Geometry check sheet. Reference: drawing and pictorial views, mm from the part's lowest x, y, z. Round coordinates to 2 decimals unless told otherwise and drop trailing zeros. Loops run counter-clockwise (first coordinate to the right, second up) from the corner with the lowest first, then second, coordinate; pieces in that order, holes last. Notation, with made-up numbers: (31, -1.5) - (70, -1.5) arc R16 cw to (70, 10.5) - close; hole circle Ø8 at (72, 68.25). An arc over 180 degrees is marked (long way). Answer as CSV lines item,"result". Start each with the question number.
1) Cross-section at D-D on y = 5.5. Record the boundary of the cut face in (x, z), and give its area (3 significant figures).
2) Draft check along X on the marked faces 1, 2 and 3. Enter one of: released by +X, released by -X, zero draft, split by the parting line, or undercut.
3) Cross-section at C-C on y = 3.25. Record the boundary of the cut face in (x, z).
4) Cross-section at B-B on z = 0.6. Record the boundary of the cut face in (x, y).
5) Cross-section at A-A on x = 4.25. Record the boundary of the cut face in (y, z).
6) Thickness scan on line 1 along X through (y, z) = (3.75, 0.45); line 2 along Y through (x, z) = (2.75, 0.3); line 3 along X through (y, z) = (4.25, 0.65). Record the ranges inside material, lowest first.
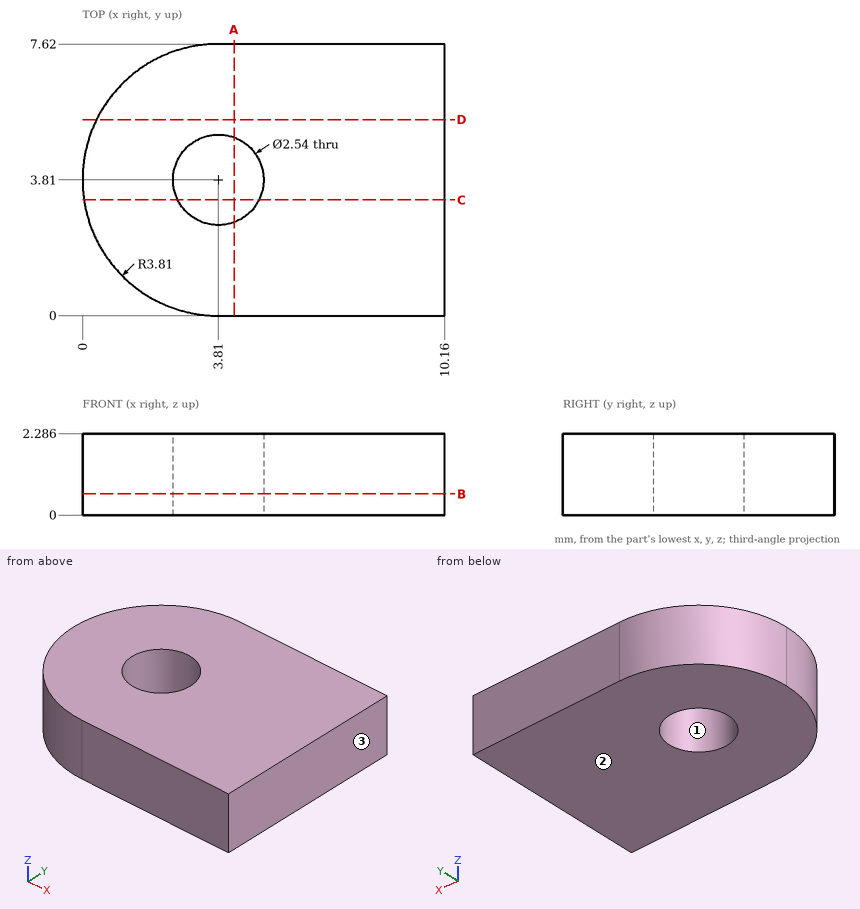
Answer block:
1,outline,"(0.4, 0) - (10.16, 0) - (10.16, 2.29) - (0.4, 2.29) - close"
1,area,"22.3 mm^2"
2,face 1,"undercut"
2,face 2,"zero draft"
2,face 3,"released by +X"
3,outline,"(0.04, 0) - (2.67, 0) - (2.67, 2.29) - (0.04, 2.29) - close; (4.95, 0) - (10.16, 0) - (10.16, 2.29) - (4.95, 2.29) - close"
4,outline,"(0, 3.81) arc R3.81 ccw to (3.81, 0) - (10.16, 0) - (10.16, 7.62) - (3.81, 7.62) arc R3.81 ccw to start; hole circle Ø2.54 at (3.81, 3.81)"
5,outline,"(0, 0) - (2.62, 0) - (2.62, 2.29) - (0, 2.29) - close; (5, 0) - (7.62, 0) - (7.62, 2.29) - (5, 2.29) - close"
6,line 1,"x = 0 to 2.54, 5.08 to 10.16"
6,line 2,"y = 0.15 to 3.11, 4.51 to 7.47"
6,line 3,"x = 0.03 to 2.62, 5 to 10.16"
